```python
from build123d import *

# Parameters (mm, degrees)
SKETCH_1_R      = 1.55
SKETCH_1_R_2    = 4
EXTRUDE_1_DEPTH = 3


with BuildPart() as part:
    # 草图1 → 凸台-拉伸1 (new body)
    with BuildSketch(Plane.XY):
        Polygon((3214.80265522, 1769.419217818), (3225.30265522, 1769.419217818), (3225.30265522, 1772.419217818), (3233.30265522, 1772.419217818), (3233.30265522, 1769.419217818), (3243.80265522, 1769.419217818), (3243.80265522, 1772.419217818), (3251.80265522, 1772.419217818), (3251.80265522, 1769.419217818), (3256.30265522, 1769.419217818), (3256.30265522, 1758.169217818), (3253.30265522, 1758.169217818), (3253.30265522, 1750.669217818), (3256.30265522, 1750.669217818), (3256.30265522, 1739.419217818), (3251.80265522, 1739.419217818), (3251.80265522, 1736.419217818), (3243.80265522, 1736.419217818), (3243.80265522, 1739.419217818), (3233.30265522, 1739.419217818), (3233.30265522, 1736.419217818), (3225.30265522, 1736.419217818), (3225.30265522, 1739.419217818), (3214.80265522, 1739.419217818), (3214.80265522, 1736.419217818), (3206.80265522, 1736.419217818), (3206.80265522, 1739.419217818), (3202.30265522, 1739.419217818), (3202.30265522, 1750.669217818), (3205.30265522, 1750.669217818), (3205.30265522, 1758.169217818), (3202.30265522, 1758.169217818), (3202.30265522, 1769.419217818), (3206.80265522, 1769.419217818), (3206.80265522, 1772.419217818), (3214.80265522, 1772.419217818), align=None)
        with Locations((3236.30265522, 1754.419217818)):
            Circle(SKETCH_1_R, mode=Mode.SUBTRACT)
        with Locations((3229.30265522, 1761.419217818)):
            Circle(SKETCH_1_R, mode=Mode.SUBTRACT)
        with Locations((3222.30265522, 1754.419217818)):
            Circle(SKETCH_1_R, mode=Mode.SUBTRACT)
        with Locations((3229.30265522, 1747.419217818)):
            Circle(SKETCH_1_R, mode=Mode.SUBTRACT)
        with Locations((3229.30265522, 1754.419217818)):
            Circle(SKETCH_1_R_2, mode=Mode.SUBTRACT)
        with Locations((3247.80265522, 1754.419217818)):
            Circle(SKETCH_1_R, mode=Mode.SUBTRACT)
        with Locations((3210.80265522, 1754.419217818)):
            Circle(SKETCH_1_R, mode=Mode.SUBTRACT)
    extrude(amount=EXTRUDE_1_DEPTH)


solid = part.part
```
Here's how the part is built. I have some questions about the finished solid (model axes, mm). A direction names the side the tool comes from. Round coordinates to 2 decimals unless told otherwise and drop trailing zeros. Loops run counter-clockwise (first coordinate to the right, second up) from the corner with the lowest first, then second, coordinate; pieces in that order, holes last. Notation, with made-up numbers: (8, 9) -> (67, 9) arc R17 ccw to (67, 34) -> close; hole circle Ø11 at (49.25, 52). An arc over 180 degrees is marked (long way). Answer as CSV lines item,"result". Start each with the question number.
1. Imagine slicing it at D-D on x = 3240.5. Write out the boundary of the cut face in (y, z).
2. If we mould it in two halves opening along Y, with no side actions, what happens to faces 1 (the face through (3227.754, 1747.487, 1.479)), 2 (the face through (3202.303, 1745, 1)), 3 (the face through (3254, 1769.419, 1))? For each: pulls with the +Y half, pulls with the -Y half, needs draft (parallel to the pull), parting line crosses it, or undercut.
3. Imagine slicing it at C-C on y = 1746.5. Write out the boundary of the cut face in (x, z), plus the area to 3 significant figures.
4. Imagine slicing it at B-B on x = 3232.5. Write out the boundary of the cut face in (y, z), plus the area to 3 significant figures.
5. For faces 4 (the face through (3251.803, 1771, 1)), 5 (the face through (3204, 1758.169, 1)), 6 (the face through (3238, 1769.419, 1)), 7 (the face through (3251.803, 1738, 1)), 8 (the face through (3214.803, 1738, 1)), which set-ups out of +Z, -Z, +X, -X, +Y, -Y let a thin tool reach every point of the face, with its end or its side?
6. Imagine slicing it at A-A on y = 1770. Write out the boundary of the cut face in (x, z).
7. I need wall thicknesses on probe 1 along X at (y, z) = (1754.5, 0.2); probe 2 along X at (y, z) = (1753.5, 0.6); probe 3 along Y at (x, z) = (3231, 1.75). Which ranges of each line are inside material? Lowest first, please. Write a range as from..to.
8. I'm going to push flat-ended pins straight in: P1, Ø1.9, axis at x = 3247.8, y = 1754.42, coming from the +Z side; P2, Ø1.5, axis at y = 1754, z = 0.5, coming from the +X side; P3, Ø0.9, axis at x = 3239.5, z = 1, coming from the +Y side; P4, Ø1.5, axis at y = 1771.5, z = 1.5, coming from the -X side. Where does each tip first touch, or does it pass through?
Solution:
1,outline,"(1739.42, 0) -> (1769.42, 0) -> (1769.42, 3) -> (1739.42, 3) -> close"
2,face 1,"undercut"
2,face 2,"needs draft"
2,face 3,"pulls with the +Y half"
3,outline,"(3202.3, 0) -> (3228.05, 0) -> (3228.05, 3) -> (3202.3, 3) -> close; (3230.55, 0) -> (3256.3, 0) -> (3256.3, 3) -> (3230.55, 3) -> close"
3,area,"155 mm²"
4,outline,"(1736.42, 0) -> (1752.02, 0) -> (1752.02, 3) -> (1736.42, 3) -> close; (1756.82, 0) -> (1772.42, 0) -> (1772.42, 3) -> (1756.82, 3) -> close"
4,area,"93.6 mm²"
5,face 4,"+Z, -Z, +X, +Y"
5,face 5,"+Z, -Z, -X"
5,face 6,"+Z, -Z, +Y"
5,face 7,"+Z, -Z, +X, -Y"
5,face 8,"+Z, -Z, -Y"
6,outline,"(3206.8, 0) -> (3214.8, 0) -> (3214.8, 3) -> (3206.8, 3) -> close; (3225.3, 0) -> (3233.3, 0) -> (3233.3, 3) -> (3225.3, 3) -> close; (3243.8, 0) -> (3251.8, 0) -> (3251.8, 3) -> (3243.8, 3) -> close"
7,probe 1,"3205.3..3209.25, 3212.35..3220.75, 3223.85..3225.3, 3233.3..3234.75, 3237.85..3246.25, 3249.35..3253.3"
7,probe 2,"3205.3..3209.55, 3212.05..3221.05, 3223.55..3225.41, 3233.2..3235.05, 3237.55..3246.55, 3249.05..3253.3"
7,probe 3,"1736.42..1750.8, 1758.04..1772.42"
8,P1,"through"
8,P2,"x = 3253.3"
8,P3,"y = 1769.42"
8,P4,"x = 3206.8"
